Can you work these out from the model? Positions are in its coordinate system, mm. Face numbers are marked on the shaded views. A direction names the side the tool comes from. Round coordinates to 2 decimals unless told otherwise and drop trailing zeros. Write each loop counter-clockwise with the first axis right and the second up, starting at its lowest first coordinate (ties: lowest second). Pieces come first, ordered by that corner, then holes. Notation, with made-up numbers: M 11,-10.5 L 31,-10.5 A26 cw 31,5.5 Z; hole C -13,48 d4. An arc over 180 degrees is marked long. Answer in a Markdown table with one row per item. Add a question column.
(1) Suppose I cut it at A-A, the plane z = -47.5. Write out the boundary of the cut face in (x, y).
(2) Suppose I cut it at C-C, the plane x = 0. Write out the boundary of the cut face in (y, z) (3 decimals).
(3) For the marked faces 1, 2 and 3, which set-ups out of +Z, -Z, +X, -X, +Y, -Y let a thin tool reach every point of the face, with its end or its side?
(4) If we mould it in two halves opening along Y, with no side actions, what happens to the marked faces 4, 5 and 6? For each: released by +Y, released by -Y, zero draft, split by the parting line, or undercut.
(5) I'm going to push flat-ended pins straight in: pin 1 (5 mm diameter, centred on x = 8.5, z = -6, fed in from +Y); pin 2 (1.5 mm diameter, centred on y = -29, z = -28, fed in from -X); pin 3 (6 mm diameter, centred on y = -25.5, z = -48, fed in from -X). Where does each tip first touch, or does it pass through?
(6) If I drill on probe 1 along Y at (x, z) = (0, 7); probe 2 along Z at (x, y) = (-25, -42.5) (3 decimals); probe 3 along Z at (x, y) = (-2, -16.5) (3 decimals), over which ranges is the centre line in solid material (lowest first)?
(7) Suppose I cut it at B-B, the plane y = -26. Write out the boundary of the cut face in (x, z) (3 decimals).
(8) Suppose I cut it at D-D, the plane x = 9. Write out the boundary of the cut face in (y, z) (1 decimal), then the cut area to 3 significant figures.
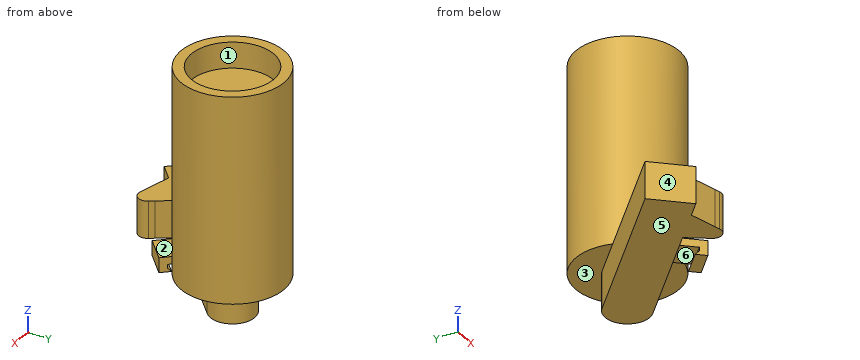
Autodesk Inventor part; units mm, degrees
ref_plane "Work Plane3" through (-4, -4, -10) normal (0, 0, -1) x (0, 1, 0)
ref_plane "Work Plane4" through (-20.0043, -85.0498, -55.625) normal (0, 0, -1) x (0, 1, 0)
ref_plane "Work Plane7" through (-4, -24.6987, -7) normal (0, 0, -1) x (0, 1, 0)
ref_plane "Work Plane3" through (-4, -4, -10) normal (0, 0, -1) x (0, 1, 0)
ref_plane "Work Plane6" through (0, 0, -10) normal (0, 0, -1) x (-1, 0, 0)
ref_plane "Work Plane4" through (-20.0043, -85.0498, -55.625) normal (0, 0, -1) x (0, 1, 0)
ref_plane "Work Plane5" through (0, 0, -55.625) normal (0, 0, -1) x (-1, 0, 0)
sketch "Sketch6" plane through (0, 0, -55.625) normal (0, 0, -1) x (-1, 0, 0)
  arc A0 (75.4786, 4.8454) -> (74.2911, 5.1636) centre (74.7523, 4.5099) ccw
  arc A1 (56.7048, 9.4732) -> (74.2911, 5.1636) centre (67.3726, 14.9684) ccw
  line L0 (55.5232, 13.0737) -> (56.7048, 9.4732)
  arc A2 (55.5232, 13.0737) -> (41.5887, -50.9456) centre (67.3725, -23.0316) ccw
  line L1 (33.4464, -59.7606) -> (41.5887, -50.9456)
  arc A3 (33.4464, -59.7606) -> (104.1015, -56.9577) centre (67.3725, -23.0316) ccw
  line L2 (112.9165, -65.0999) -> (104.1015, -56.9577)
  arc A4 (112.9165, -65.0999) -> (124.3718, -47.4258) centre (67.3725, -23.0316) ccw
  line L3 (113.3397, -42.7043) -> (124.3718, -47.4258)
  arc A5 (113.3397, -42.7043) -> (116.0567, -34.4268) centre (67.3725, -23.0316) ccw
  arc A6 (116.0567, -34.4268) -> (112.8612, -32.4083) centre (114.1093, -33.971) ccw
  arc A7 (103.4777, -34.8812) -> (112.8612, -32.4083) centre (105.3725, -23.0317) ccw
  line L4 (99.8772, -33.6995) -> (103.4777, -34.8812)
  arc A8 (95.5677, -16.1132) -> (99.8772, -33.6995) centre (105.3725, -23.0317) ccw
  arc A9 (95.5677, -16.1132) -> (95.2495, -14.9257) centre (94.9141, -15.652) ccw
  arc A10 (88.3311, -2.9425) -> (95.2495, -14.9257) centre (100.2815, -4.0317) ccw
  arc A11 (88.3311, -2.9425) -> (87.4618, -2.0732) centre (87.5344, -2.8699) ccw
  arc A12 (75.4786, 4.8454) -> (87.4618, -2.0732) centre (86.3726, 9.8773) ccw
  circle A13 centre (67.3725, -23.0316) radius 18
  line L5 (41.5887, -50.9456) -> (4.0711, -16.2912)
  line L6 (33.4464, -59.7606) -> (-4.0711, -25.1062)
  line L7 (-32.6275, -120.0316) -> (-32.6275, 19.9684)
  line L8 (-32.6275, 19.9684) -> (137.3725, 19.9684)
  line L9 (33.4464, -59.7606) -> (41.5887, -50.9456)
  circle A14 centre (0, -20.6987) radius 6
  arc A15 (18.8962, -53.3592) -> (15.9689, -49.5949) centre (16.8391, -51.9385) ccw
  line L10 (18.8962, -53.3592) -> (18.0411, -54.5974)
  arc A16 (18.0411, -54.5974) -> (20.7197, -58.4396) centre (20.0982, -56.0181) ccw
  line L11 (20.7197, -58.4396) -> (22.1832, -58.064)
  arc A17 (24.7026, -62.1127) -> (22.1832, -58.064) centre (22.8047, -60.4856) ccw
  line L12 (24.7026, -62.1127) -> (10.325, -78.8833)
  arc A18 (-4.734, -57.2821) -> (10.325, -78.8833) centre (0, -70.0316) ccw
  line L13 (-4.734, -57.2821) -> (15.9689, -49.5949)
  circle A19 centre (0, -70.0316) radius 5.6
  line L14 (18.8962, -53.3592) -> (21.8639, -49.062)
  line L15 (22.1832, -58.064) -> (29.5601, -56.1709)
extrude "Extrusion5" add sketch "Sketch6" against normal blind 10 contours L1 L6 A14 L5 | A14 | L15 L11 A16 L10 L14 L6
sketch "Sketch7" plane through (0, -20.6987, -45.625) normal (0, 0, 1) x (1, 0, 0)
  circle A0 centre (0, 0) radius 11.2
  circle A1 centre (0, 0) radius 14
  point P0 (0, 20.6987)
  dimension "d14" = 22.4
  dimension "d15" = 28
ref_plane "Work Plane7" through (-4, -24.6987, -7) normal (0, 0, -1) x (0, 1, 0)
extrude "Extrusion6" add sketch "Sketch7" along normal blind 48.625 contours A0 | A1
sketch "Sketch8" plane through (0, -20.6987, 3) normal (0, 0, 1) x (1, 0, 0)
  circle A0 centre (0, 0) radius 4
  circle A1 centre (0, 0) radius 11.2
  circle A2 centre (0, 0) radius 14
  point P0 (0, 20.6987)
  dimension "d18" = 8
  dimension "d19" = 22.4
extrude "Extrusion7" add sketch "Sketch8" along normal blind 7 contours A2
ref_plane "Work Plane8" through (-11.409, -39.4049, -55.625) normal (-0.7345804, -0.6785217, 0) x (0, 0, 1)
sketch "Sketch10" plane through (-11.409, -39.4049, -55.625) normal (-0.7345804, -0.6785217, 0) x (0, 0, 1)
  line L0 (0, 0) -> (0, 12)
  line L1 (0, 12) -> (10, 12)
  line L2 (10, 12) -> (10, 0)
  line L3 (10, 0) -> (0, 0)
  line L4 (0, 0) -> (0, 12)
  line L5 (2, 0) -> (2, -8)
  line L6 (2, -8) -> (7, -8)
  line L7 (7, -8) -> (7, -4)
  line L8 (7, -4) -> (5, -6)
  line L9 (5, -6) -> (4, -6)
  line L10 (4, -6) -> (4, 0)
  line L11 (6, 0) -> (6, -8)
  line L12 (6, -8) -> (1, -8)
  line L13 (1, -8) -> (1, -4)
  line L14 (1, -4) -> (3, -6)
  line L15 (3, -6) -> (4, -6)
  point P0 (55.625, 21.2048)
  point P1 (6, 0)
  point P2 (2, -5)
  point P3 (6, -8)
  dimension "d23" = 8
  dimension "d24" = 5
  dimension "d25" = 4
  dimension "d26" = 45
  dimension "d27" = 2
  dimension "d28" = 2
  dimension "d29" = 2
extrude "Extrusion8" add sketch "Sketch10" along normal mid plane 8 contours L3 L11 L8 L9 L10 | L14 L15 L9 L8 L11 L6 L5
properties part number "ReverserClicker"
Calculated:
| question | item | result |
|---|---|---|
| 1 | outline | M -41.59,-50.95 L -33.45,-59.76 L -29.56,-56.17 L -22.18,-58.06 L -20.72,-58.44 A2.5 ccw -18.04,-54.6 L -18.9,-53.36 L -21.86,-49.06 L 4.07,-25.11 A6 ccw -4.07,-16.29 Z |
| 2 | outline | M -34.699,-45.625 L -28.867,-45.625 L -28.867,-55.625 L -14.699,-55.625 L -14.699,-45.625 L -6.699,-45.625 L -6.699,10 L -9.499,10 L -9.499,3 L -31.899,3 L -31.899,10 L -34.699,10 Z |
| 3 | face 1 | +Z |
| 3 | face 2 | +Z, +X, -Y |
| 3 | face 3 | -Z |
| 4 | face 4 | released by -Y |
| 4 | face 5 | zero draft |
| 4 | face 6 | undercut |
| 5 | pin 1 | y = -8.05 |
| 5 | pin 2 | x = -11.79 |
| 5 | pin 3 | x = -17.29 |
| 6 | probe 1 | -34.7 to -31.9, -9.5 to -6.7 |
| 6 | probe 2 | -55.625 to -45.625 |
| 6 | probe 3 | -55.625 to 3 |
| 7 | outline | M -14.582,-55.625 L 3.103,-55.625 L 3.103,-45.625 L 12.957,-45.625 L 12.957,10 L 9.866,10 L 9.866,3 L -9.866,3 L -9.866,10 L -12.957,10 L -12.957,-45.625 L -14.582,-45.625 Z |
| 8 | outline | M -31.4,-45.6 L -10,-45.6 L -10,10 L -14,10 L -14,3 L -27.4,3 L -27.4,10 L -31.4,10 Z |
| 8 | area | 1,100 mm² |
